The drawing under review shows one solid part. Ordinate dimensions are in mm from its lowest x, y, z. A direction names the side the tool comes from. Give positions to 0.01 mm unless a question says otherwise; leave off trailing zeros. Order: outer loops, then holes, each group sorted by start corner. A loop starts at its lowest first (then second) coordinate and runs counter-clockwise, first axis right, second up. Notation, with made-up numbers: (62, 57) -> (80, 57) arc R14 cw to (80, 67) -> close; hole circle Ø7 at (-17.75, 79). An arc over 180 degrees is marked (long way). One line per item, written item: value.
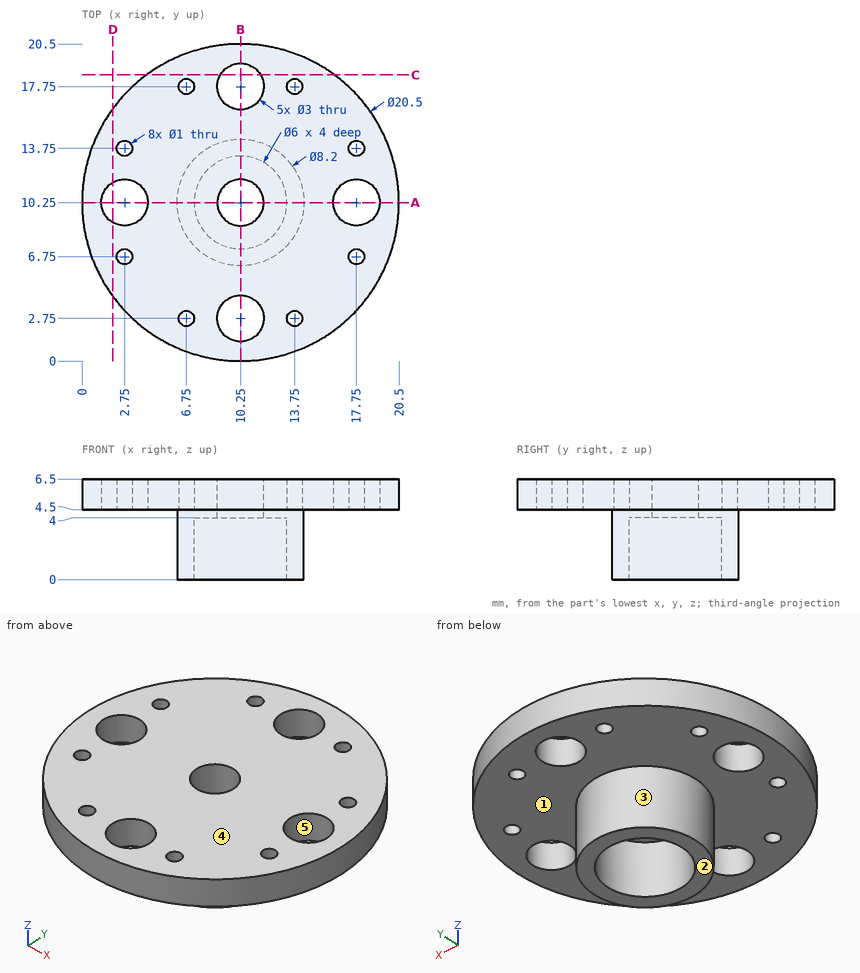
Item 1: Draft analysis for pull direction X (two halves, no side actions). For the marked faces 3, 4 and 5, state which applies: pulls with the +X half, pulls with the -X half, needs draft (parallel to the pull), parting line crosses it, or undercut.
Returned:
face 3: parting line crosses it
face 4: needs draft
face 5: undercut
Item 2: Add section C-C on y = 18.5. Give the boundary of the cut face in (x, z).
Returned:
outline: (4.17, 4.5) -> (8.95, 4.5) -> (8.95, 6.5) -> (4.17, 6.5) -> close; (11.55, 4.5) -> (16.33, 4.5) -> (16.33, 6.5) -> (11.55, 6.5) -> close
Item 3: Clearance check with flat-ended pins moving along their axes: P1, Ø1, axis at x = 8.5, z = 4.5, coming from the -Y side; P2, Ø3, axis at x = 9, z = 2.5, coming from the -Y side; P3, Ø3, axis at x = 11, y = 11.5, coming from the -Z side; P4, Ø10, axis at x = 10, y = 8, coming from the -Z side. State where each tip first meets the part, or that it passes through.
Returned:
P1: y = 0.08
P2: y = 6.15
P3: z = 4
P4: z = 0
Item 4: Add section A-A on y = 10.25. Give the boundary of the cut face in (x, z), plus the area to 3 significant figures.
Returned:
outline: (0, 4.5) -> (1.25, 4.5) -> (1.25, 6.5) -> (0, 6.5) -> close; (4.25, 4.5) -> (6.15, 4.5) -> (6.15, 0) -> (7.25, 0) -> (7.25, 4) -> (8.75, 4) -> (8.75, 6.5) -> (4.25, 6.5) -> close; (11.75, 4) -> (13.25, 4) -> (13.25, 0) -> (14.35, 0) -> (14.35, 4.5) -> (16.25, 4.5) -> (16.25, 6.5) -> (11.75, 6.5) -> close; (19.25, 4.5) -> (20.5, 4.5) -> (20.5, 6.5) -> (19.25, 6.5) -> close
area: 34.4 mm²
Item 5: To check wall thickness, follow line 1 along Y through (x, z) = (10.25, 5); line 2 along X through (y, z) = (6.75, 6.1); line 3 along Y through (x, z) = (17.75, 5.3). State the ranges of each line that lie inside material, in increasing order. Write a range as from..to.
Returned:
line 1: 0..1.25, 4.25..8.75, 11.75..16.25, 19.25..20.5
line 2: 0.62..2.25, 3.25..17.25, 18.25..19.88
line 3: 3.26..6.25, 7.25..8.75, 11.75..13.25, 14.25..17.24
Item 6: Machinability: for the marked faces 1 and 2, which of the approach directions +Z, -Z, +X, -X, +Y, -Y give a long, thin tool a straight path to every point of the face, cutting with its end or side? Answer none if there is none.
Returned:
face 1: -Z
face 2: -Z, +X, -X, +Y, -Y
